```python
from build123d import *

# Parameters (mm, degrees)
SKETCH_1_W      = 52
SKETCH_1_H      = 52
EXTRUDE_1_DEPTH = 3
SKETCH_2_W      = 52
SKETCH_2_H      = 52
SKETCH_2_R      = 1.5
SKETCH_2_R_2    = 8.8
EXTRUDE_2_DEPTH = 3


with BuildPart() as part:
    # 草圖1 → 填料-伸長1 (new body)
    with BuildSketch(Plane(origin=(0, 0, 0), x_dir=(1, 0, 0), z_dir=(0, 1, 0))):
        Rectangle(SKETCH_1_W, SKETCH_1_H)
        with BuildLine():
            Line((-15.5, 20.6), (-13.5, 20.6))
            ThreePointArc((-13.5, 20.6), (-10.4, 17.5), (-13.5, 14.4))
            Line((-13.5, 14.4), (-15.5, 14.4))
            ThreePointArc((-15.5, 14.4), (-18.6, 17.5), (-15.5, 20.6))
        make_face(mode=Mode.SUBTRACT)
        with BuildLine():
            Line((15.5, 20.6), (13.5, 20.6))
            ThreePointArc((13.5, 20.6), (10.4, 17.5), (13.5, 14.4))
            Line((13.5, 14.4), (15.5, 14.4))
            ThreePointArc((15.5, 14.4), (18.6, 17.5), (15.5, 20.6))
        make_face(mode=Mode.SUBTRACT)
        with BuildLine():
            Line((15.5, -20.6), (13.5, -20.6))
            ThreePointArc((13.5, -20.6), (10.4, -17.5), (13.5, -14.4))
            Line((13.5, -14.4), (15.5, -14.4))
            ThreePointArc((15.5, -14.4), (18.6, -17.5), (15.5, -20.6))
        make_face(mode=Mode.SUBTRACT)
        with BuildLine():
            Line((-15.5, -20.6), (-13.5, -20.6))
            ThreePointArc((-13.5, -20.6), (-10.4, -17.5), (-13.5, -14.4))
            Line((-13.5, -14.4), (-15.5, -14.4))
            ThreePointArc((-15.5, -14.4), (-18.6, -17.5), (-15.5, -20.6))
        make_face(mode=Mode.SUBTRACT)
    extrude(amount=EXTRUDE_1_DEPTH)

    # 草圖2 → 填料-伸長2 (add)
    with BuildSketch(Plane(origin=(0, 0, -26), x_dir=(-1, 0, 0), z_dir=(0, 0, -1))):
        with Locations((0, 26)):
            Rectangle(SKETCH_2_W, SKETCH_2_H)
        with Locations((-14.5, 28)):
            Circle(SKETCH_2_R, mode=Mode.SUBTRACT)
        with Locations((14.5, 28)):
            Circle(SKETCH_2_R, mode=Mode.SUBTRACT)
        with Locations((0, 28)):
            Circle(SKETCH_2_R_2, mode=Mode.SUBTRACT)
    extrude(amount=EXTRUDE_2_DEPTH)


solid = part.part
```
Check sheet for the modelled part. Datum: model origin and axes. Units: mm. A direction names the side the tool comes from. Coordinates: 2 decimals unless noted, no trailing zeros. Order: outer loops, then holes, each group sorted by start corner. A loop starts at its lowest first (then second) coordinate and runs counter-clockwise, first axis right, second up. Notation, with made-up numbers: M 34,34 L 42,34 A26 cw 42,62 Z; hole C 23,50.25 d5. An arc over 180 degrees is marked long. Write each question's results on one line, items separated by ' | '. Start each with the question number.
1. Mould release check, pull along X, two halves, no side actions. Record for faces 1 (the face through (14, 1, -14.4)), 2 (the face through (-26, 2.8, -9.5)), 3 (the face through (6, 21, -29)): +X half, -X half, draft (parallel to the pull), parting line (faces both ways), or undercut.
2. Cross-section at D-D on x = 14.5. Record the cut outline in (y, z).
3. Cross-section at C-C on z = 17.5. Record the cut outline in (x, y), and give its area (3 significant figures).
4. Access from +Z, -Z, +X, -X, +Y, -Y to the whole of each face (thin tool, end or side, straight path). Record for faces 4 (the face through (14, 1, 14.4)), 5 (the face through (0, 3, 0)), 6 (the face through (-14.305, 29.487, -27.479)).
5. Cross-section at A-A on x = 0. Record the cut outline in (y, z).
6. Cross-section at B-B on y = 28. Record the cut outline in (x, z), and give its area (3 significant figures).
7. Material ranges on probe 1 along Y at (x, z) = (0, -28.3); probe 2 along Z at (x, y) = (24.5, 17); probe 3 along Y at (x, z) = (24, -17.5), recorded low to high.
8. Go/stop test with flat-tipped pins: P1, Ø20, axis at x = 0, y = 28, coming from the +Z side; P2, Ø3, axis at x = -2.5, z = 5, coming from the +Y side. Record where each tip stops, or that it passes through.
Checks:
1) face 1: undercut | face 2: -X half | face 3: draft
2) outline: M 0,-29 L 26.5,-29 L 26.5,-26 L 3,-26 L 3,-20.6 L 0,-20.6 Z; M 0,-14.4 L 3,-14.4 L 3,14.4 L 0,14.4 Z; M 0,20.6 L 3,20.6 L 3,26 L 0,26 Z; M 29.5,-29 L 52,-29 L 52,-26 L 29.5,-26 Z
3) outline: M -26,0 L -18.6,0 L -18.6,3 L -26,3 Z; M -10.4,0 L 10.4,0 L 10.4,3 L -10.4,3 Z; M 18.6,0 L 26,0 L 26,3 L 18.6,3 Z | area: 107 mm²
4) face 4: +Y, -Y | face 5: +Z, +X, -X, +Y | face 6: +Z, -Z
5) outline: M 0,-29 L 19.2,-29 L 19.2,-26 L 3,-26 L 3,26 L 0,26 Z; M 36.8,-29 L 52,-29 L 52,-26 L 36.8,-26 Z
6) outline: M -26,-29 L -16,-29 L -16,-26 L -26,-26 Z; M -13,-29 L -8.8,-29 L -8.8,-26 L -13,-26 Z; M 8.8,-29 L 13,-29 L 13,-26 L 8.8,-26 Z; M 16,-29 L 26,-29 L 26,-26 L 16,-26 Z | area: 85.2 mm²
7) probe 1: y = 0 to 19.2, 36.8 to 52 | probe 2: z = -29 to -26 | probe 3: y = 0 to 3
8) P1: stops at z = -26 | P2: stops at y = 3
